```python
from build123d import *

# Parameters (mm, degrees)
SKETCH1_W           = 100
SKETCH1_H           = 120
SKETCH1_R           = 2.5
SKETCH1_W_2         = 5
SKETCH1_H_2         = 40
BOSS_EXTRUDE1_DEPTH = 4
CHAMFER1_SIZE       = 10


with BuildPart() as part:
    # Sketch1 → Boss-Extrude1 (new, symmetric)
    with BuildSketch(Plane.XY):
        with Locations((0, 60)):
            Rectangle(SKETCH1_W, SKETCH1_H)
        with Locations((-42, 6.66986634)):
            Circle(SKETCH1_R, mode=Mode.SUBTRACT)
        with Locations((-42, 34.66986634)):
            Circle(SKETCH1_R, mode=Mode.SUBTRACT)
        with Locations((-10.5, 112)):
            Circle(SKETCH1_R, mode=Mode.SUBTRACT)
        with Locations((-10.5, 84)):
            Circle(SKETCH1_R, mode=Mode.SUBTRACT)
        with Locations(Location((10.5, 84, 0), (0, 0, 180))):
            Circle(SKETCH1_R, mode=Mode.SUBTRACT)
        with Locations(Location((10.5, 112, 0), (0, 0, 180))):
            Circle(SKETCH1_R, mode=Mode.SUBTRACT)
        with Locations((-21, 6.66986634)):
            Circle(SKETCH1_R, mode=Mode.SUBTRACT)
        with Locations((-21, 34.66986634)):
            Circle(SKETCH1_R, mode=Mode.SUBTRACT)
        with Locations(Location((21, 34.66986634, 0), (0, 0, 180))):
            Circle(SKETCH1_R, mode=Mode.SUBTRACT)
        with Locations(Location((21, 6.66986634, 0), (0, 0, 180))):
            Circle(SKETCH1_R, mode=Mode.SUBTRACT)
        with Locations(Location((42, 34.66986634, 0), (0, 0, 180))):
            Circle(SKETCH1_R, mode=Mode.SUBTRACT)
        with Locations(Location((42, 6.66986634, 0), (0, 0, 180))):
            Circle(SKETCH1_R, mode=Mode.SUBTRACT)
        with Locations((37.5, 95)):
            Rectangle(SKETCH1_W_2, SKETCH1_H_2, mode=Mode.SUBTRACT)
        with Locations((-37.5, 95)):
            Rectangle(SKETCH1_W_2, SKETCH1_H_2, mode=Mode.SUBTRACT)
    extrude(amount=BOSS_EXTRUDE1_DEPTH, both=True)

    # Chamfer1
    chamfer1_edges = [part.edges().sort_by_distance(p)[0] for p in [
        (-50, 120, 0),
        (50, 120, 0),
    ]]
    chamfer(chamfer1_edges, length=CHAMFER1_SIZE)


solid = part.part
```
Design review of the part built by this model. Coordinates are the model's own, in mm. A direction names the side the tool comes from. Give positions to 0.01 mm unless a question says otherwise; leave off trailing zeros. Order: outer loops, then holes, each group sorted by start corner. A loop starts at its lowest first (then second) coordinate and runs counter-clockwise, first axis right, second up. Notation, with made-up numbers: (66, 14.5) - (75, 14.5) arc R19 ccw to (75, 50.5) - close; hole circle Ø4 at (36, 58). An arc over 180 degrees is marked (long way). Use a Markdown table: item, result. Add a question column.
(1) Machinability: for faces 1 (the face through (-1, 61, 4)), 2 (the face through (-38, 75, 0)), which of the approach directions +Z, -Z, +X, -X, +Y, -Y give a long, thin tool a straight path to every point of the face, cutting with its end or side? Answer none if there is none.
(2) Wall thickness on probe 1 along Y at (x, z) = (-10.5, -2.25); probe 2 along X at (y, z) = (81, -1); probe 3 along Y at (x, z) = (21, 1.5): over which ranges is each line inside the solid? List them lowest first. Write a range as [from, to].
(3) Add section A-A on x = -10.5. Give the boundary of the cut face in (y, z).
(4) Mouldability with a two-part tool opening along X and no side actions: class faces 3 (the face through (-45, 115, 0)), 4 (the face through (-40.66, 36.78, -0.06)), 5 (the face through (-1, 120, 0)) as +X half, -X half, draft (parallel to the pull), parting line (faces both ways), or undercut.
(5) Add section B-B on y = 102.5. Give the boundary of the cut face in (x, z).
(6) Clearance check with a flat-ended pin moving along its axis: P1, Ø3, axis at x = 21, y = 6.67, coming from the -Z side. State where the tip first meets the part, or that it passes through.
(7) Add section C-C on y = 84. Give the boundary of the cut face in (x, z), then the cut area to 3 significant figures.
(8) Add section D-D on z = -2.75. Give the number of separate pieces and of enclosed holes in the cut face, then the cut area to 3 significant figures.
Report:
| question | item | result |
|---|---|---|
| 1 | face 1 | +Z, +X, -X, +Y, -Y |
| 1 | face 2 | +Z, -Z |
| 2 | probe 1 | y = [0, 81.5], [86.5, 109.5], [114.5, 120] |
| 2 | probe 2 | x = [-50, -40], [-35, 35], [40, 50] |
| 2 | probe 3 | y = [0, 4.17], [9.17, 32.17], [37.17, 120] |
| 3 | outline | (0, -4) - (81.5, -4) - (81.5, 4) - (0, 4) - close; (86.5, -4) - (109.5, -4) - (109.5, 4) - (86.5, 4) - close; (114.5, -4) - (120, -4) - (120, 4) - (114.5, 4) - close |
| 4 | face 3 | -X half |
| 4 | face 4 | undercut |
| 4 | face 5 | draft |
| 5 | outline | (-50, -4) - (-40, -4) - (-40, 4) - (-50, 4) - close; (-35, -4) - (35, -4) - (35, 4) - (-35, 4) - close; (40, -4) - (50, -4) - (50, 4) - (40, 4) - close |
| 6 | P1 | passes through |
| 7 | outline | (-50, -4) - (-40, -4) - (-40, 4) - (-50, 4) - close; (-35, -4) - (-13, -4) - (-13, 4) - (-35, 4) - close; (-8, -4) - (8, -4) - (8, 4) - (-8, 4) - close; (13, -4) - (35, -4) - (35, 4) - (13, 4) - close; (40, -4) - (50, -4) - (50, 4) - (40, 4) - close |
| 7 | area | 640 mm² |
| 8 | separate pieces | 1 |
| 8 | enclosed holes | 14 |
| 8 | area | 11,300 mm² |
